```python
from build123d import *

# Parameters (mm, degrees)
F0_W     = 14.03
F0_H     = 5
F0_W_2   = 13.9
F0_H_2   = 25
F0_W_3   = 9.3
F0_W_4   = 7.09
F0_H_3   = 50
F1_DEPTH = 4
F2_DEPTH = 6


with BuildPart() as f1:
    # F0 (on Top) → F1 (new body)
    with BuildSketch(Plane.XY):
        with Locations((-23.265, 27.5)):
            Rectangle(F0_W, F0_H)
        with Locations((0, -27.5)):
            Rectangle(F0_W_2, F0_H)
        with Locations((46.595, -27.5)):
            Rectangle(F0_W, F0_H)
        Polygon((-62.91, 25), (-62.91, 30), (-80, 30), (-80, -30), (-62.91, -30), (-62.91, -25), (-70, -25), (-70, 25), align=None)
        with Locations((23.265, -12.5)):
            Rectangle(F0_W, F0_H_2)
        with Locations((58.26, -27.5)):
            Rectangle(F0_W_3, F0_H)
        with Locations((34.93, 27.5)):
            Rectangle(F0_W_3, F0_H)
        with Locations((-11.6, -27.5)):
            Rectangle(F0_W_3, F0_H)
        with Locations((-66.455, 0)):
            Rectangle(F0_W_4, F0_H_3)
        with Locations((23.265, 27.5)):
            Rectangle(F0_W, F0_H)
        with Locations((66.455, 0)):
            Rectangle(F0_W_4, F0_H_3)
        with Locations((-58.26, 27.5)):
            Rectangle(F0_W_3, F0_H)
        with Locations((46.595, 27.5)):
            Rectangle(F0_W, F0_H)
        with Locations((-46.595, 27.5)):
            Rectangle(F0_W, F0_H)
        Polygon((80, -30), (80, 30), (62.91, 30), (62.91, 25), (70, 25), (70, -25), (62.91, -25), (62.91, -30), align=None)
        with Locations((-34.93, 27.5)):
            Rectangle(F0_W_3, F0_H)
        with Locations((58.26, 27.5)):
            Rectangle(F0_W_3, F0_H)
        with Locations((11.6, 27.5)):
            Rectangle(F0_W_3, F0_H)
        with Locations((0, 27.5)):
            Rectangle(F0_W_2, F0_H)
        with Locations((-23.265, -27.5)):
            Rectangle(F0_W, F0_H)
        with Locations((-11.6, 27.5)):
            Rectangle(F0_W_3, F0_H)
        with Locations((23.265, -27.5)):
            Rectangle(F0_W, F0_H)
        with Locations((-34.93, -27.5)):
            Rectangle(F0_W_3, F0_H)
        with Locations((-46.595, 0)):
            Rectangle(F0_W, F0_H_3)
        with Locations((23.265, 12.5)):
            Rectangle(F0_W, F0_H_2)
        Polygon((6.95, 0), (6.95, 25), (-6.95, 25), (-6.95, -25), (6.95, -25), align=None)
        with Locations((34.93, -27.5)):
            Rectangle(F0_W_3, F0_H)
        with Locations((-46.595, -27.5)):
            Rectangle(F0_W, F0_H)
        with Locations((46.595, 12.5)):
            Rectangle(F0_W, F0_H_2)
        with Locations((46.595, -12.5)):
            Rectangle(F0_W, F0_H_2)
        with Locations((-58.26, -27.5)):
            Rectangle(F0_W_3, F0_H)
        with Locations((-23.265, 0)):
            Rectangle(F0_W, F0_H_3)
        with Locations((11.6, -27.5)):
            Rectangle(F0_W_3, F0_H)
        with Locations((-58.26, 0)):
            Rectangle(F0_W_3, F0_H_3)
        with Locations((-34.93, 0)):
            Rectangle(F0_W_3, F0_H_3)
        with Locations((-11.6, 0)):
            Rectangle(F0_W_3, F0_H_3)
        Polygon((16.25, -25), (16.25, 0), (11.6, 0), (6.95, 0), (6.95, -25), align=None)
        Polygon((16.25, 0), (16.25, 25), (6.95, 25), (6.95, 0), (11.6, 0), align=None)
        Polygon((39.58, 0), (39.58, 25), (30.28, 25), (30.28, 0), (34.93, 0), align=None)
        Polygon((62.91, -25), (62.91, 25), (53.61, 25), (53.61, 0), (53.61, -25), align=None)
        Polygon((39.58, -25), (39.58, 0), (34.93, 0), (30.28, 0), (30.28, -25), align=None)
    extrude(amount=-F1_DEPTH)

    # F0 (on Top) → F2 (join)
    with BuildSketch(Plane.XY):
        Polygon((-62.91, 25), (-62.91, 30), (-80, 30), (-80, -30), (-62.91, -30), (-62.91, -25), (-70, -25), (-70, 25), align=None)
        with Locations((-46.595, 27.5)):
            Rectangle(F0_W, F0_H)
        with Locations((-46.595, -27.5)):
            Rectangle(F0_W, F0_H)
        with Locations((-23.265, -27.5)):
            Rectangle(F0_W, F0_H)
        with Locations((-23.265, 27.5)):
            Rectangle(F0_W, F0_H)
        with Locations((0, 27.5)):
            Rectangle(F0_W_2, F0_H)
        with Locations((0, -27.5)):
            Rectangle(F0_W_2, F0_H)
        with Locations((23.265, -27.5)):
            Rectangle(F0_W, F0_H)
        with Locations((23.265, 27.5)):
            Rectangle(F0_W, F0_H)
        with Locations((46.595, 27.5)):
            Rectangle(F0_W, F0_H)
        with Locations((46.595, -27.5)):
            Rectangle(F0_W, F0_H)
        Polygon((80, -30), (80, 30), (62.91, 30), (62.91, 25), (70, 25), (70, -25), (62.91, -25), (62.91, -30), align=None)
    extrude(amount=F2_DEPTH)


solid = f1.part
```
The listing builds one solid part. Answer for the finished solid, in the listing's coordinates (mm). A direction names the side the tool comes from. Coordinates: 2 decimals unless noted, no trailing zeros. Loops run counter-clockwise (first coordinate to the right, second up) from the corner with the lowest first, then second, coordinate; pieces in that order, holes last. Notation, with made-up numbers: (13, 87.25) - (68, 87.25) arc R33 ccw to (68, 122.25) - close; hole circle Ø6 at (67.5, 53.5). An arc over 180 degrees is marked (long way). Write item = value, one per line.
1) Find the intervals of material crossed by line 1 along X through (y, z) = (2, 2); line 2 along Y through (x, z) = (-44.5, 0.5); line 3 along Z through (x, y) = (10.5, 23), in increasing order.
Responses:
line_1 = -80 to -70, 70 to 80
line_2 = -30 to -25, 25 to 30
line_3 = -4 to 0
2) Section B-B (y = 1) is taken. Determine the outline of the cut face in (x, z), plus the area to 3 significant figures.
Responses:
outline = (-80, -4) - (80, -4) - (80, 6) - (70, 6) - (70, 0) - (-70, 0) - (-70, 6) - (-80, 6) - close
area = 760 mm^2
3) Section C-C (z = 2.5) is taken. Count the separate pieces of the cut face and the enclosed holes in it, plus the area to 3 significant figures.
Responses:
separate_pieces = 12
enclosed_holes = 0
area = 2,040 mm^2
4) Section D-D (x = -14.5) is taken. Determine the outline of the cut face in (y, z), plus the area to 3 significant figures.
Responses:
outline = (-30, -4) - (30, -4) - (30, 0) - (-30, 0) - close
area = 240 mm^2
5) Section A-A (x = 22) is taken. Determine the outline of the cut face in (y, z).
Responses:
outline = (-30, -4) - (30, -4) - (30, 6) - (25, 6) - (25, 0) - (-25, 0) - (-25, 6) - (-30, 6) - close
6) Which of the six approach directions +Z, -Z, +X, -X, +Y, -Y give full straight-line access (tool end or side, diameter ignored) to faces 1 (the face through (0, 28, 6)), 2 (the face through (6.95, 27, 3)), 3 (the face through (70, 0, 3))?
Responses:
face_1 = +Z, +X, -X, +Y, -Y
face_2 = +Z, +Y, -Y
face_3 = +Z
7) Determine the mould class of faces 4 (the face through (-62.91, 27, 3)), 5 (the face through (-6.95, -28, 3)), 6 (the face through (-23, -27, 6)), 7 (the face through (-80, 0, 1)) for opening direction X: pulls with the +X half, pulls with the -X half, needs draft (parallel to the pull), parting line crosses it, or undercut.
Responses:
face_4 = undercut
face_5 = undercut
face_6 = needs draft
face_7 = pulls with the -X half
